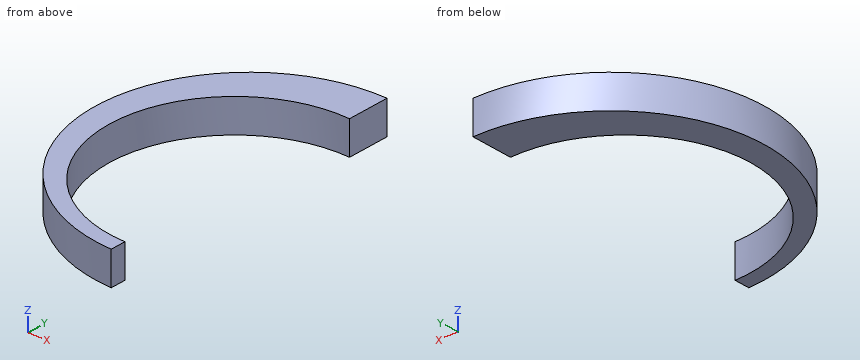
```python
from build123d import *

# Parameters (mm, degrees)
F0_R     = 116.287792
F1_DEPTH = 25
F2_R     = 94.758514
F3_DEPTH = 25.001
F5_DEPTH = 25.001


with BuildPart() as f1:
    # F0 (on Top) → F1 (new body)
    with BuildSketch(Plane.XY):
        with Locations((-180.245414, -20.226402)):
            Circle(F0_R)
    extrude(amount=F1_DEPTH)

    # F2 (on face) → F3 (cut, through all)
    with BuildSketch(Plane.XY.offset(25)):
        with Locations((-182.132989, -30.261295)):
            Circle(F2_R)
    extrude(amount=-F3_DEPTH, mode=Mode.SUBTRACT)

    # F4 (on face) → F5 (cut, through all)
    with BuildSketch(Plane.XY.offset(25)):
        Polygon((-180.245414, 124.963261), (-180.245414, -20.226402), (-180.245414, -167.464018), (-41.918594, -167.464018), (-41.918594, 124.963261), align=None)
    extrude(amount=-F5_DEPTH, mode=Mode.SUBTRACT)


solid = f1.part
```
CAD build for the part. Positions are in the model's coordinates, mm. Coordinates: 2 decimals unless noted, no trailing zeros. Order: outer loops, then holes, each group sorted by start corner. A loop starts at its lowest first (then second) coordinate and runs counter-clockwise, first axis right, second up. Notation, with made-up numbers: (28, 77) -> (57, 77) arc R21 ccw to (57, 111) -> close; hole circle Ø7 at (-24, -1.75). An arc over 180 degrees is marked (long way). Use one line per item in the form item = value. Start each with the question number.
1) Drill centre lines: L1, parallel to Y at x = -216.5, z = 5.25; L2, parallel to Y at x = -217.5, z = 8.25; L3, parallel to X at y = 2, z = 21. Where is each one in solid material? Low to high. Write a range as [from, to].
2) Band-saw the part on A-A on x = -258. Give the cut face in (y, z), then the cut area to 3 significant figures.
3) Drop flat-ended pins along their axis: pin 1 (3 mm diameter, centred on y = -30, z = 10, fed in from +X); pin 2 (6 mm diameter, centred on x = -197, z = 22, fed in from -Y); pin 3 (5 mm diameter, centred on y = -53, z = 15.5, fed in from +X); pin 4 (5 mm diameter, centred on x = -257, y = -83.5, fed in from +Z). Give the stop position or say it passes through.
4) Band-saw the part on D-D on y = 13.5. Give the cut face in (x, z), then the cut area to 3 significant figures.
5) Band-saw the part on C-C on x = -232. Give the cut face in (y, z), then the cut area to 3 significant figures.
Entries:
q1.L1 = [-130.72, -118.57], [58.05, 90.27]
q1.L2 = [-130.39, -118.17], [57.65, 89.93]
q1.L3 = [-294.39, -271.23]
q2.outline = (-106.7, 0) -> (-87.04, 0) -> (-87.04, 25) -> (-106.7, 25) -> close; (26.51, 0) -> (66.24, 0) -> (66.24, 25) -> (26.51, 25) -> close
q2.area = 1,480 mm2
q3.pin_1 = -276.88
q3.pin_2 = -135.7
q3.pin_3 = -273.47
q3.pin_4 = through
q4.outline = (-291.54, 0) -> (-266.18, 0) -> (-266.18, 25) -> (-291.54, 25) -> close
q4.area = 634 mm2
q5.outline = (-124.36, 0) -> (-110.84, 0) -> (-110.84, 25) -> (-124.36, 25) -> close; (50.31, 0) -> (83.91, 0) -> (83.91, 25) -> (50.31, 25) -> close
q5.area = 1,180 mm2
